from build123d import *

# Parameters (mm, degrees)
ESQUISSE1_W      = 5
ESQUISSE1_H      = 5
EXTRUSION1_DEPTH = 5
ESQUISSE2_R      = 2.4
EXTRUSION2_DEPTH = 4
EXTRUSION2_TAPER = 10
ESQUISSE3_R      = 2.4
EXTRUSION3_DEPTH = 4
EXTRUSION3_TAPER = 10
ESQUISSE4_R      = 2.4
EXTRUSION4_DEPTH = 4
EXTRUSION4_TAPER = 10
ESQUISSE5_R      = 2.2
EXTRUSION5_DEPTH = 5
EXTRUSION5_TAPER = 10
ESQUISSE6_R      = 2.2
EXTRUSION6_DEPTH = 5
EXTRUSION6_TAPER = 10
ESQUISSE7_R      = 2.2
EXTRUSION7_DEPTH = 5
EXTRUSION7_TAPER = 10


with BuildPart() as part:
    # Esquisse1 → Extrusion1 (new body)
    with BuildSketch(Plane.XY):
        with Locations((-16.829438543, -10.768512898)):
            Rectangle(ESQUISSE1_W, ESQUISSE1_H)
    extrude(amount=EXTRUSION1_DEPTH)

    # Esquisse2 → Extrusion2 (add)
    with BuildSketch(Plane(origin=(-14.329438543, 0, 0), x_dir=(0, 0, -1), z_dir=(1, 0, 0))):
        with Locations((-2.5, -10.768512898)):
            Circle(ESQUISSE2_R)
    extrude(amount=EXTRUSION2_DEPTH, taper=EXTRUSION2_TAPER)

    # Esquisse3 → Extrusion3 (add)
    with BuildSketch(Plane(origin=(0, -8.268512898, 0), x_dir=(-1, 0, 0), z_dir=(0, 1, 0))):
        with Locations((16.829438543, 2.5)):
            Circle(ESQUISSE3_R)
    extrude(amount=EXTRUSION3_DEPTH, taper=EXTRUSION3_TAPER)

    # Esquisse4 → Extrusion4 (add)
    with BuildSketch(Plane.ZY.offset(19.329438543)):
        with Locations((2.5, -10.768512898)):
            Circle(ESQUISSE4_R)
    extrude(amount=EXTRUSION4_DEPTH, taper=EXTRUSION4_TAPER)

    # Esquisse5 → Extrusion5 (add)
    with BuildSketch(Plane.ZY.offset(23.329438543)):
        with Locations((2.5, -10.768512898)):
            Circle(ESQUISSE5_R)
    extrude(amount=EXTRUSION5_DEPTH, taper=EXTRUSION5_TAPER)

    # Esquisse6 → Extrusion6 (add)
    with BuildSketch(Plane(origin=(0, -4.268512898, 0), x_dir=(-1, 0, 0), z_dir=(0, 1, 0))):
        with Locations((16.829438543, 2.5)):
            Circle(ESQUISSE6_R)
    extrude(amount=EXTRUSION6_DEPTH, taper=EXTRUSION6_TAPER)

    # Esquisse7 → Extrusion7 (add)
    with BuildSketch(Plane(origin=(-10.329438543, 0, 0), x_dir=(0, 0, -1), z_dir=(1, 0, 0))):
        with Locations((-2.5, -10.768512898)):
            Circle(ESQUISSE7_R)
    extrude(amount=EXTRUSION7_DEPTH, taper=EXTRUSION7_TAPER)


solid = part.part
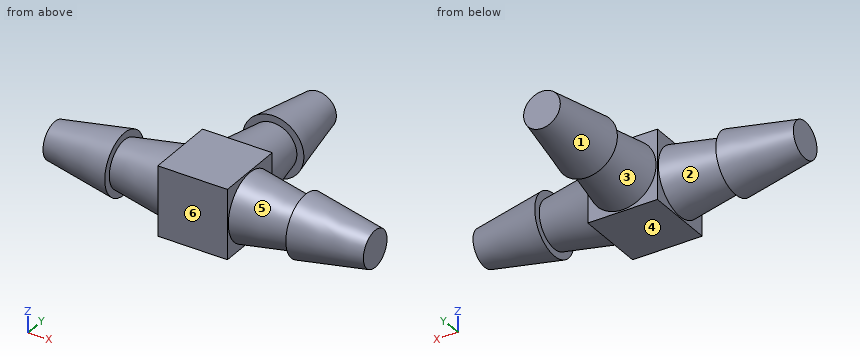
Could you check a few things on this model? Use its own coordinates, in mm. Face numbers are marked on the shaded views. A direction names the side the tool comes from. Give positions to 0.01 mm unless a question says otherwise; leave off trailing zeros. Loops run counter-clockwise (first coordinate to the right, second up) from the corner with the lowest first, then second, coordinate; pieces in that order, holes last. Notation, with made-up numbers: M 10.5,-15.75 L 35.5,-15.75 A19 cw 35.5,-7.75 Z; hole C 56,84.5 d2. An arc over 180 degrees is marked long. Answer as a JSON object with one key per item and string values.
Q1. For P1, Ø1.5, axis at x = -18.5, y = -11, coming from the -Z side; P2, Ø2, axis at x = -19.5, y = -6.5, coming from the -Z side, each with a flat end and sliding along its axis, tell me the tip position at first contact or that it passes through.
Values found:
{"P1": "stops at z = 0", "P2": "stops at z = 1.22"}
Q2. Suppose I cut it at A-A, the plane x = -21. List the corners of the cut face in (y, z) for me, plus the area to 3 significant figures.
Values found:
{"outline": "C -10.77,2.5 d4.21", "area": "13.9 mm²"}
Q3. For the marked faces 5 and 6, which set-ups out of +Z, -Z, +X, -X, +Y, -Y let a thin tool reach every point of the face, with its end or its side?
Values found:
{"face 5": "none", "face 6": "+Z, -Z, +X, -X, -Y"}
Q4. Suppose I cut it at B-B, the plane y = -5.25. List the corners of the cut face in (x, z) for me.
Values found:
{"outline": "C -16.83,2.5 d3.74"}
Q5. If I drill on probe 1 along X at (y, z) = (-3.75, 1.7); probe 2 along Z at (x, y) = (-27.5, -10.5); probe 3 along X at (y, z) = (-7, 2.25), over which ranges is the centre line in solid material (lowest first)? Write a range as [from, to].
Values found:
{"probe 1": "x = [-18.78, -14.88]", "probe 2": "z = [1.06, 3.94]", "probe 3": "x = [-18.99, -14.67]"}
Q6. If we mould it in two halves opening along Y, with no side actions, what happens to the marked faces 1, 2, 3 and 4? For each: pulls with the +Y half, pulls with the -Y half, needs draft (parallel to the pull), parting line crosses it, or undercut.
Values found:
{"face 1": "pulls with the +Y half", "face 2": "parting line crosses it", "face 3": "undercut", "face 4": "needs draft"}
